CAD build for the part. Positions are in the model's coordinates, mm. A direction names the side the tool comes from. Give positions to 0.01 mm unless a question says otherwise; leave off trailing zeros. Write each loop counter-clockwise with the first axis right and the second up, starting at its lowest first coordinate (ties: lowest second). Pieces come first, ordered by that corner, then holes. Notation, with made-up numbers: (-6, 44) - (25, 44) arc R20 ccw to (25, 54) - close; hole circle Ø6 at (14.25, 61). An arc over 180 degrees is marked (long way). Put each result on its own line as item: value. Start each with the question number.
1. Cut at C-C on y = 5.1. List the corners of the cut face in (x, z).
2. Drop flat-ended pins along their axis: pin 1 (1.5 mm diameter, centred on x = -38.5, y = 5, fed in from -Z); pin 2 (1.5 mm diameter, centred on y = 4.5, z = -46, fed in from +X); pin 3 (2.5 mm diameter, centred on x = -60.5, y = 4.5, fed in from +Z). Give the stop position or say it passes through.
3. Cut at A-A on z = -44.5. List the corners of the cut face in (x, y).
4. Tool access for faces 1 (the cylindrical face through (-85, 5, -64)), 2 (the flat face through (-45, 4, -6)), 3 (the flat face through (-46, 4, -4)), 4 (the flat face through (-86, 4, -21)), 5 (the cylindrical face through (-84.99, 5.43, -38.1)): list every direction of +Z, -Z, +X, -X, +Y, -Y with a clear straight run to the whole face (end or side of a thin tool).
5. Cut at B-B on x = -52. List the corners of the cut face in (y, z).
6. Wall check: line 1 (X direction, y = 3.9, z = -30); line 2 (Z direction, x = -41.5, y = 5.35); line 3 (Y direction, x = -22, z = -16.5). Give the ranges that are in metal, low to high.
7. Mould opens along X. For faces 6 (the flat face through (0, 1, -35)), 7 (the cylindrical face through (-85, 5, -6)), 8 (the flat face through (-46, 1, 0)), 9 (the cylindrical face through (-8, 5, -7)) say: +X half, -X half, draft (parallel to the pull), parting line (faces both ways), or undercut.
8. Cut at D-D on z = -5. List the corners of the cut face in (x, y).
from build123d import *

# Parameters (mm, degrees)
ESBO_O1_W                = 90
ESBO_O1_H                = 70
ESBO_O1_W_2              = 82
ESBO_O1_H_2              = 62
ESBO_O1_W_3              = 78
ESBO_O1_H_3              = 58
RESSALTO_EXTRUS_O1_DEPTH = 3
ESBO_O1_3_W              = 82
ESBO_O1_3_H              = 62
ESBO_O1_3_W_2            = 78
ESBO_O1_3_H_2            = 58
RESSALTO_EXTRUS_O2_DEPTH = 6
FILETE1_R                = 3
FILETE2_R                = 5
CORTE_EXTRUS_O1_REACH    = 113.05
ESBO_O2_W                = 5
ESBO_O2_H                = 3
FILETE3_R                = 2


with BuildPart() as part:
    # Esbo_o1 → Ressalto-extrus_o1 (new body)
    # profile 1 of 3: a face of its own
    with BuildSketch(Plane(origin=(0, 0, 0), x_dir=(1, 0, 0), z_dir=(0, 1, 0))):
        with Locations((-45, 35)):
            Rectangle(ESBO_O1_W, ESBO_O1_H)
        with Locations((-45, 35)):
            Rectangle(ESBO_O1_W_2, ESBO_O1_H_2, mode=Mode.SUBTRACT)
    # profile 2 of 3: a face of its own
    with BuildSketch(Plane(origin=(0, 0, 0), x_dir=(1, 0, 0), z_dir=(0, 1, 0))):
        with Locations((-45, 35)):
            Rectangle(ESBO_O1_W_2, ESBO_O1_H_2)
        with Locations((-45, 35)):
            Rectangle(ESBO_O1_W_3, ESBO_O1_H_3, mode=Mode.SUBTRACT)
    # profile 3 of 3: a face of its own
    with BuildSketch(Plane(origin=(0, 0, 0), x_dir=(1, 0, 0), z_dir=(0, 1, 0))):
        with Locations((-45, 35)):
            Rectangle(ESBO_O1_W_3, ESBO_O1_H_3)
    extrude(amount=RESSALTO_EXTRUS_O1_DEPTH)

    # Esbo_o1_3 → Ressalto-extrus_o2 (add)
    with BuildSketch(Plane(origin=(0, 0, 0), x_dir=(1, 0, 0), z_dir=(0, 1, 0))):
        with Locations((-45, 35)):
            Rectangle(ESBO_O1_3_W, ESBO_O1_3_H)
        with Locations((-45, 35)):
            Rectangle(ESBO_O1_3_W_2, ESBO_O1_3_H_2, mode=Mode.SUBTRACT)
    extrude(amount=RESSALTO_EXTRUS_O2_DEPTH)

    # Filete1
    filete1_edges = [part.edges().sort_by_distance(p)[0] for p in [
        (-90, 1.5, -70),
        (0, 1.5, -70),
        (0, 1.5, 0),
        (-90, 1.5, 0),
    ]]
    fillet(filete1_edges, radius=FILETE1_R)

    # Filete2
    filete2_edges = [part.edges().sort_by_distance(p)[0] for p in [
        (-86, 4.5, -4),
        (-4, 4.5, -4),
        (-4, 4.5, -66),
        (-6, 4.5, -64),
        (-6, 4.5, -6),
        (-84, 4.5, -6),
        (-84, 4.5, -64),
        (-86, 4.5, -66),
    ]]
    fillet(filete2_edges, radius=FILETE2_R)

    # Esbo_o2 → Corte-extrus_o1 (cut, up to next)
    with BuildSketch(Plane.ZY.offset(86), mode=Mode.PRIVATE) as corte_extrus_o1_sk1:
        with Locations((-35, 4.5)):
            Rectangle(ESBO_O2_W, ESBO_O2_H)
    corte_extrus_o1_tool1 = extrude(corte_extrus_o1_sk1.sketch, amount=-CORTE_EXTRUS_O1_REACH, mode=Mode.PRIVATE) & part.part
    add(corte_extrus_o1_tool1.solids().sort_by_distance((-86, 4.5, -35))[0], mode=Mode.SUBTRACT)

    # Filete3
    filete3_edges = [part.edges().sort_by_distance(p)[0] for p in [
        (-85, 6, -32.5),
        (-85, 6, -37.5),
    ]]
    fillet(filete3_edges, radius=FILETE3_R)


solid = part.part
Report:
1. outline: (-86, -61) arc R5 ccw to (-81, -66) - (-9, -66) arc R5 ccw to (-4, -61) - (-4, -9) arc R5 ccw to (-9, -4) - (-81, -4) arc R5 ccw to (-86, -9) - (-86, -32.17) - (-84, -32.17) - (-84, -11) arc R5 cw to (-79, -6) - (-11, -6) arc R5 cw to (-6, -11) - (-6, -59) arc R5 cw to (-11, -64) - (-79, -64) arc R5 cw to (-84, -59) - (-84, -37.83) - (-86, -37.83) - close
2. pin 1: stops at z = -66
2. pin 2: stops at x = -4
2. pin 3: stops at z = -4
3. outline: (-90, 0) - (0, 0) - (0, 3) - (-4, 3) - (-4, 6) - (-6, 6) - (-6, 3) - (-84, 3) - (-84, 6) - (-86, 6) - (-86, 3) - (-90, 3) - close
4. face 1: -Z, -X, +Y
4. face 2: +Y
4. face 3: +Z, +X, -X, +Y
4. face 4: +Z, -Z, -X, +Y
4. face 5: -X, +Y
5. outline: (0, -70) - (3, -70) - (3, -66) - (6, -66) - (6, -64) - (3, -64) - (3, -6) - (6, -6) - (6, -4) - (3, -4) - (3, 0) - (0, 0) - close
6. line 1: x = -86 to -84, -6 to -4
6. line 2: z = -66 to -64, -6 to -4
6. line 3: y = 0 to 3
7. face 6: +X half
7. face 7: -X half
7. face 8: draft
7. face 9: undercut
8. outline: (-90, 0) - (0, 0) - (0, 3) - (-6, 3) - (-6, 6) - (-84, 6) - (-84, 3) - (-90, 3) - close
